```python
from build123d import *

# Parameters (mm, degrees)
SKETCH_1_W                   = 90
SKETCH_1_H                   = 90
EXTRUDE_2_DEPTH              = 65.5
SKETCH_2_R                   = 42.5
CUT_EXTRUDE_1_DEPTH          = 3
SKETCH_3_R                   = 18
EXTRUDE_3_DEPTH              = 7.5
SKETCH_4_R                   = 7.5
EXTRUDE_4_DEPTH              = 33.5
EXTRUDE_5_REACH              = 166.05
HOLE_WIZARD_M6_1_D           = 5
HOLE_WIZARD_M6_1_DEPTH       = 17
HOLE_WIZARD_M6_1_CSINK_D     = 6.05
HOLE_WIZARD_M6_1_CSINK_ANGLE = 90
HOLE_WIZARD_M6_1_TIP         = 1.502151548
FILLET_1_R                   = 10
HOLE_WIZARD_M6_2_D           = 5
HOLE_WIZARD_M6_2_DEPTH       = 17
HOLE_WIZARD_M6_2_CSINK_D     = 6.05
HOLE_WIZARD_M6_2_CSINK_ANGLE = 90
HOLE_WIZARD_M6_2_TIP         = 1.502151548


with BuildPart() as part:
    # 草图1 → 凸台-拉伸2 (new body)
    with BuildSketch(Plane.XY):
        with Locations((45, -45)):
            Rectangle(SKETCH_1_W, SKETCH_1_H)
    extrude(amount=EXTRUDE_2_DEPTH)

    # 草图2 → 切除-拉伸1 (cut)
    with BuildSketch(Plane.XY.offset(65.5)):
        with Locations((45, -45)):
            Circle(SKETCH_2_R)
    extrude(amount=-CUT_EXTRUDE_1_DEPTH, mode=Mode.SUBTRACT)

    # 草图3 → 凸台-拉伸3 (add)
    with BuildSketch(Plane.XY.offset(62.5)):
        with Locations((45, -27)):
            Circle(SKETCH_3_R)
    extrude(amount=EXTRUDE_3_DEPTH)

    # 草图4 → 凸台-拉伸4 (add)
    with BuildSketch(Plane.XY.offset(70)):
        with Locations((45, -27)):
            Circle(SKETCH_4_R)
    extrude(amount=EXTRUDE_4_DEPTH)

    # 草图5 → 凸台-拉伸5 (add, up to next)
    with BuildSketch(Plane.XY.offset(103.5), mode=Mode.PRIVATE) as extrude_5_sk1:
        with BuildLine():
            Line((42.5, -19.928932188), (42.5, -17.928932188))
            Line((42.5, -17.928932188), (47.5, -17.928932188))
            Line((47.5, -17.928932188), (47.5, -19.928932188))
            ThreePointArc((47.5, -19.928932188), (45, -19.5), (42.5, -19.928932188))
        make_face()
    extrude_5_tool1 = extrude(extrude_5_sk1.sketch, amount=-EXTRUDE_5_REACH, mode=Mode.PRIVATE) - part.part
    add(extrude_5_tool1.solids().sort_by_distance((45, -18.789851, 103.5))[0])

    # M6 螺纹孔1
    with Locations(Plane.XY.offset(65.5)):
        with Locations((9.644660941, -9.644660941), (80.355339059, -9.644660941), (9.644660941, -80.355339059), (80.355339059, -80.355339059)):
            CounterSinkHole(HOLE_WIZARD_M6_1_D / 2, HOLE_WIZARD_M6_1_CSINK_D / 2, depth=HOLE_WIZARD_M6_1_DEPTH, counter_sink_angle=HOLE_WIZARD_M6_1_CSINK_ANGLE)
            with Locations((0, 0, -(HOLE_WIZARD_M6_1_DEPTH + HOLE_WIZARD_M6_1_TIP / 2))):  # 118° drill point
                Cone(0, HOLE_WIZARD_M6_1_D / 2, HOLE_WIZARD_M6_1_TIP, mode=Mode.SUBTRACT)

    # 圆角1
    fillet_1_edges = [part.edges().sort_by_distance(p)[0] for p in [
        (0, 0, 32.75),
        (90, 0, 32.75),
        (90, -90, 32.75),
        (0, -90, 32.75),
    ]]
    fillet(fillet_1_edges, radius=FILLET_1_R)

    # M6 螺纹孔2
    with Locations(Plane(origin=(0, 0, 0), x_dir=(-1, 0, 0), z_dir=(0, 0, -1))):
        with Locations((-9.602967378, -80.397032622), (-80.31359627, -9.68640373), (-9.602967378, -9.602967378), (-80.31359627, -80.31359627)):
            CounterSinkHole(HOLE_WIZARD_M6_2_D / 2, HOLE_WIZARD_M6_2_CSINK_D / 2, depth=HOLE_WIZARD_M6_2_DEPTH, counter_sink_angle=HOLE_WIZARD_M6_2_CSINK_ANGLE)
            with Locations((0, 0, -(HOLE_WIZARD_M6_2_DEPTH + HOLE_WIZARD_M6_2_TIP / 2))):  # 118° drill point
                Cone(0, HOLE_WIZARD_M6_2_D / 2, HOLE_WIZARD_M6_2_TIP, mode=Mode.SUBTRACT)


solid = part.part
```
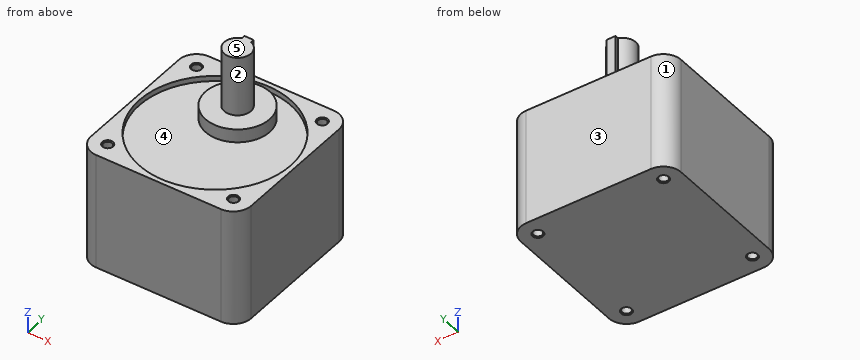
Here's how the part is built. I have some questions about the finished solid (model axes, mm). Face numbers are marked on the shaded views. A direction names the side the tool comes from. Round coordinates to 2 decimals unless told otherwise and drop trailing zeros. Order: outer loops, then holes, each group sorted by start corner. A loop starts at its lowest first (then second) coordinate and runs counter-clockwise, first axis right, second up. Notation, with made-up numbers: (18.5, -14.5) -> (69.5, -14.5) arc R26 cw to (69.5, 15.5) -> close; hole circle Ø3 at (-28, 57). An arc over 180 degrees is marked (long way). Use a Markdown table: item, result. Add a question column.
(1) Suppose I cut it at A-A, the plane x = 45. Please give me the cut outline in (y, z), and give its area (3 significant figures).
(2) For pin 1 Ø4 at (x, y) = (19, -57.5) entering from +Z; pin 2 Ø12 at (x, y) = (35.5, -12) entering from +Z; pin 3 Ø3 at (x, y) = (80.36, -80.36) entering from -Z, each with a flat end and sliding along its axis, tell me the tip position at first contact or that it passes through.
(3) I need wall thicknesses on line 1 along Y through (x, z) = (45, 63.65); line 2 along Y through (x, z) = (10, 5); line 3 along Z through (x, y) = (34, -11). Which ranges of each line are inside material? Lowest first, please.
(4) If we mould it in two halves opening along Y, with no side actions, what happens to the marked faces 3, 4 and 5? For each: released by +Y, released by -Y, zero draft, split by the parting line, or undercut.
(5) Suppose I cut it at C-C, the plane z = 13. Please give me the cut outline in (x, y).
(6) For the marked faces 1 and 2, which set-ups out of +Z, -Z, +X, -X, +Y, -Y let a thin tool reach every point of the face, with its end or its side?
(7) Suppose I cut it at B-B, the plane y = -27. Please give me the cut outline in (x, z), and give its area (3 significant figures).
(8) Suppose I cut it at D-D, the plane x = 69. Please give me the cut outline in (y, z), and give its area (3 significant figures).
Verdict:
| question | item | result |
|---|---|---|
| 1 | outline | (-90, 0) -> (0, 0) -> (0, 65.5) -> (-2.5, 65.5) -> (-2.5, 62.5) -> (-9, 62.5) -> (-9, 70) -> (-17.93, 70) -> (-17.93, 103.5) -> (-34.5, 103.5) -> (-34.5, 70) -> (-45, 70) -> (-45, 62.5) -> (-87.5, 62.5) -> (-87.5, 65.5) -> (-90, 65.5) -> close |
| 1 | area | 6,470 mm2 |
| 2 | pin 1 | z = 62.5 |
| 2 | pin 2 | z = 70 |
| 2 | pin 3 | z = 17.56 |
| 3 | line 1 | -90 to -87.5, -45 to -9, -2.5 to 0 |
| 3 | line 2 | -90 to -82.87, -77.93 to -12.07, -7.13 to 0 |
| 3 | line 3 | 0 to 62.5 |
| 4 | face 3 | released by +Y |
| 4 | face 4 | undercut |
| 4 | face 5 | zero draft |
| 5 | outline | (0, -80) arc R10 ccw to (10, -90) -> (80, -90) arc R10 ccw to (90, -80) -> (90, -10) arc R10 ccw to (80, 0) -> (10, 0) arc R10 ccw to (0, -10) -> close; hole circle Ø5 at (9.6, -80.4); hole circle Ø5 at (9.6, -9.6); hole circle Ø5 at (80.31, -80.31); hole circle Ø5 at (80.31, -9.69) |
| 6 | face 1 | +Z, -Z, -X, +Y |
| 6 | face 2 | +Z |
| 7 | outline | (0, 0) -> (90, 0) -> (90, 65.5) -> (83.5, 65.5) -> (83.5, 62.5) -> (63, 62.5) -> (63, 70) -> (52.5, 70) -> (52.5, 103.5) -> (37.5, 103.5) -> (37.5, 70) -> (27, 70) -> (27, 62.5) -> (6.5, 62.5) -> (6.5, 65.5) -> (0, 65.5) -> close |
| 7 | area | 6,440 mm2 |
| 8 | outline | (-90, 0) -> (0, 0) -> (0, 65.5) -> (-9.93, 65.5) -> (-9.93, 62.5) -> (-80.07, 62.5) -> (-80.07, 65.5) -> (-90, 65.5) -> close |
| 8 | area | 5,680 mm2 |
